Read the model definition and answer for the solid it produces. Units are mm, in the model's axes. Face numbers are marked on the shaded views. A direction names the side the tool comes from. Give positions to 0.01 mm unless a question says otherwise; leave off trailing zeros. Loops run counter-clockwise (first coordinate to the right, second up) from the corner with the lowest first, then second, coordinate; pieces in that order, holes last. Notation, with made-up numbers: (27, 80) - (31, 80) arc R13 cw to (31, 103) - close; hole circle Ø2 at (-2.5, 6.5). An arc over 180 degrees is marked (long way). Put each result on its own line as item: value. Start each with the question number.
1. Consider L1, parallel to Y at x = -8, z = 17.5; L2, parallel to Y at x = 17, z = 20.5; L3, parallel to X at y = 32, z = 5. Determine where each line is inside the solid, lowest interval first. Write a range as from..to.
2. A cutting plane is placed at C-C, the plane y = -9. Determine the outline of the cut face in (x, z), plus the area to 3 significant figures.
3. For a pull along Y with two mould halves and no side action, classify the marked faces 1, 2, 3 and 4 as released by +Y, released by -Y, zero draft, split by the parting line, or undercut.
4. Given pin 1 Ø2.5 at (x, y) = (-11, 4.5) entering from +Z; pin 2 Ø4 at (y, z) = (46, 10) entering from +X; pin 3 Ø8 at (x, z) = (-11.5, 3) entering from +Y; pin 4 Ø5 at (y, z) = (-9.5, 11.5) entering from -X, each flat-ended and moving along its own axis, determine where each tip first touches the part or whether it passes through.
5. A cutting plane is placed at A-A, the plane z = 5. Count the separate pieces of the cut face and the enclosed holes in it, plus the area to 3 significant figures.
6. A cutting plane is placed at B-B, the plane y = 46. Determine the outline of the cut face in (x, z), plus the area to 3 significant figures.
7. For the marked faces 5, 6 and 7, determine the directions among +Z, -Z, +X, -X, +Y, -Y from which every point of the face is accessible in a straight line to the end or side of a thin tool.
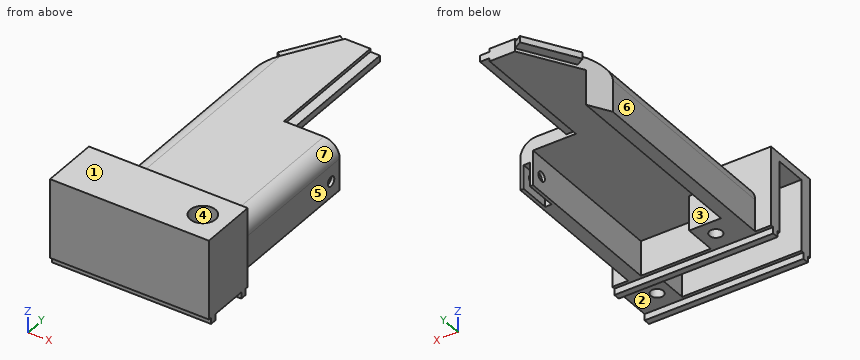
```python
from build123d import *

# Parameters (mm, degrees)
SKETCH1_W                = 40
SKETCH1_H                = 30
BOSS_EXTRUDE1_DEPTH      = 90
SHELL1_T                 = -4
FILLET1_R                = 5
CUT_EXTRUDE1_DEPTH       = 94.407708461
CUT_EXTRUDE1_DEPTH_BACK  = 94.407708461
CUT_EXTRUDE2_DEPTH       = 94.407708461
CUT_EXTRUDE2_DEPTH_BACK  = 94.407708461
SKETCH3_W                = 17.5
SKETCH3_H                = 40
SKETCH5_W                = 2
SKETCH5_H                = 40
BOSS_EXTRUDE2_DEPTH      = 3
SKETCH6_W                = 2
SKETCH6_H                = 18
BOSS_EXTRUDE3_DEPTH      = 3
SKETCH8_W                = 50
SKETCH8_H                = 50
BOSS_EXTRUDE4_DEPTH      = 18
SKETCH10_W               = 45
SKETCH10_H               = 10
CUT_EXTRUDE4_DEPTH       = 37.5
BOSS_EXTRUDE5_REACH      = 103.502
SKETCH15_W               = 10
SKETCH15_H               = 10
CUT_EXTRUDE8_DEPTH       = 103.988587343
CUT_EXTRUDE8_DEPTH_BACK  = 103.988587343
SKETCH20_R               = 2
SKETCH21_R               = 4
CUT_EXTRUDE9_DEPTH       = 5
SKETCH23_W               = 2
SKETCH23_H               = 15
CUT_EXTRUDE10_DEPTH      = 10
CUT_EXTRUDE11_START      = -10
SKETCH24_R               = 1.5
CUT_EXTRUDE11_DEPTH      = 116.031657717
CUT_EXTRUDE12_DEPTH      = 99.140965569
CUT_EXTRUDE12_DEPTH_BACK = 99.140965569
SKETCH27_W               = 50
SKETCH27_H               = 25
SKETCH29_W               = 50
SKETCH29_H               = 2
BOSS_EXTRUDE6_DEPTH      = 2
SKETCH30_W               = 50
SKETCH30_H               = 2
BOSS_EXTRUDE7_DEPTH      = 2
CUT_EXTRUDE13_DEPTH      = 99.66939304
CUT_EXTRUDE13_DEPTH_BACK = 99.66939304
SKETCH31_R               = 2
SKETCH32_R               = 4
CUT_EXTRUDE14_DEPTH      = 15


with BuildPart() as part:
    # Sketch1 → Boss-Extrude1 (new body)
    with BuildSketch(Plane(origin=(0, 0, 0), x_dir=(1, 0, 0), z_dir=(0, 1, 0))):
        Rectangle(SKETCH1_W, SKETCH1_H)
    extrude(amount=BOSS_EXTRUDE1_DEPTH)

    # Shell1
    shell1_openings = [part.faces().sort_by_distance(p)[0] for p in [
        (0, 90, 0),
        (0, 0, 0),
    ]]
    offset(amount=SHELL1_T, openings=shell1_openings, kind=Kind.INTERSECTION)

    # Fillet1
    fillet1_edges = [part.edges().sort_by_distance(p)[0] for p in [
        (20, 45, 15),
        (-20, 45, 15),
        (-20, 45, -15),
        (20, 45, -15),
    ]]
    fillet(fillet1_edges, radius=FILLET1_R)

    # Sketch2 → Cut-Extrude1 (cut, two sides: drawn at the far end of the back side and taken through both)
    with BuildSketch(Plane.XY.offset(-CUT_EXTRUDE1_DEPTH_BACK)):
        Polygon((-5.5, 90), (-20, 66), (-20, 90), align=None)
    extrude(amount=CUT_EXTRUDE1_DEPTH + CUT_EXTRUDE1_DEPTH_BACK, mode=Mode.SUBTRACT)

    # Sketch3 → Cut-Extrude2 (cut, two sides: drawn at the far end of the back side and taken through both)
    with BuildSketch(Plane.XY.offset(-CUT_EXTRUDE2_DEPTH_BACK)):
        with Locations((11.25, 70)):
            Rectangle(SKETCH3_W, SKETCH3_H)
    extrude(amount=CUT_EXTRUDE2_DEPTH + CUT_EXTRUDE2_DEPTH_BACK, mode=Mode.SUBTRACT)

    # Sketch5 → Boss-Extrude2 (add)
    with BuildSketch(Plane(origin=(2.5, 0, 0), x_dir=(0, 0, -1), z_dir=(1, 0, 0))):
        with Locations((-13, 70)):
            Rectangle(SKETCH5_W, SKETCH5_H)
    boss_extrude2 = extrude(amount=BOSS_EXTRUDE2_DEPTH)

    # Mirror1: Boss-Extrude2 across plane
    add(boss_extrude2.mirror(Plane.XY))

    # Sketch6 → Boss-Extrude3 (add)
    with BuildSketch(Plane(origin=(-43.86391097, 26.501112878, 0), x_dir=(0, 0, 1), z_dir=(-0.8559155419457906, 0.5171156399255814, 0))):
        with Locations((-13, 65.188262756)):
            Rectangle(SKETCH6_W, SKETCH6_H)
    boss_extrude3 = extrude(amount=BOSS_EXTRUDE3_DEPTH)

    # Mirror2: Boss-Extrude3 across plane
    add(boss_extrude3.mirror(Plane.XY))

    # Sketch8 → Boss-Extrude4 (add)
    with BuildSketch(Plane(origin=(0, 0, 0), x_dir=(1, 0, 0), z_dir=(0, 1, 0))):
        Rectangle(SKETCH8_W, SKETCH8_H)
    extrude(amount=-BOSS_EXTRUDE4_DEPTH)

    # Sketch10 → Cut-Extrude4 (cut)
    with BuildSketch(Plane.ZY.offset(25)):
        with Locations((0, -9)):
            Rectangle(SKETCH10_W, SKETCH10_H)
    extrude(amount=-CUT_EXTRUDE4_DEPTH, mode=Mode.SUBTRACT)

    # Sketch15 → Boss-Extrude5 (add, up to next)
    with BuildSketch(Plane.XY.offset(-11), mode=Mode.PRIVATE) as boss_extrude5_sk1:
        with Locations((-11, 5)):
            Rectangle(SKETCH15_W, SKETCH15_H)
    boss_extrude5_tool1 = extrude(boss_extrude5_sk1.sketch, amount=BOSS_EXTRUDE5_REACH, mode=Mode.PRIVATE) - part.part
    add(boss_extrude5_tool1.solids().sort_by_distance((-11, 5, -11))[0])

    # Sketch20 → Cut-Extrude8 (cut, two sides: drawn at the far end of the back side and taken through both)
    with BuildSketch(Plane(origin=(0, 0, -15), x_dir=(-1, 0, 0), z_dir=(0, 0, -1)).offset(-CUT_EXTRUDE8_DEPTH_BACK)):
        with Locations((11, 5)):
            Circle(SKETCH20_R)
    extrude(amount=CUT_EXTRUDE8_DEPTH + CUT_EXTRUDE8_DEPTH_BACK, mode=Mode.SUBTRACT)

    # Sketch21 → Cut-Extrude9 (cut)
    with BuildSketch(Plane(origin=(0, 0, -15), x_dir=(-1, 0, 0), z_dir=(0, 0, -1))):
        with Locations((11, 5)):
            Circle(SKETCH21_R)
    cut_extrude9 = extrude(amount=-CUT_EXTRUDE9_DEPTH, mode=Mode.SUBTRACT)

    # Mirror3: Cut-Extrude9 across plane
    add(cut_extrude9.mirror(Plane.XY), mode=Mode.SUBTRACT)

    # Sketch23 → Cut-Extrude10 (cut)
    with BuildSketch(Plane(origin=(0, 50, 0), x_dir=(1, 0, 0), z_dir=(0, 1, 0))):
        with Locations((17.949489743, 0)):
            Rectangle(SKETCH23_W, SKETCH23_H)
    extrude(amount=-CUT_EXTRUDE10_DEPTH, mode=Mode.SUBTRACT)

    # Sketch24 → Cut-Extrude11 (cut)
    with BuildSketch(Plane(origin=(20, 0, 0), x_dir=(0, 0, -1), z_dir=(1, 0, 0)).offset(CUT_EXTRUDE11_START)):
        with Locations(Location((-5, 46, 0), (0, 0, 180))):
            Circle(SKETCH24_R)
    cut_extrude11 = extrude(amount=CUT_EXTRUDE11_DEPTH, mode=Mode.SUBTRACT)

    # Mirror4: Cut-Extrude11 across plane
    add(cut_extrude11.mirror(Plane.XY), mode=Mode.SUBTRACT)

    # Sketch27 → Cut-Extrude12 (cut, two sides: drawn at the far end of the back side and taken through both)
    with BuildSketch(Plane(origin=(0, 0, 0), x_dir=(1, 0, 0), z_dir=(0, 1, 0)).offset(-CUT_EXTRUDE12_DEPTH_BACK)):
        with Locations((0, 12.5)):
            Rectangle(SKETCH27_W, SKETCH27_H)
    extrude(amount=CUT_EXTRUDE12_DEPTH + CUT_EXTRUDE12_DEPTH_BACK, mode=Mode.SUBTRACT)

    # Sketch29 → Boss-Extrude6 (add)
    with BuildSketch(Plane(origin=(0, 0, 0), x_dir=(-1, 0, 0), z_dir=(0, 0, -1))):
        with Locations((0, -2)):
            Rectangle(SKETCH29_W, SKETCH29_H)
    extrude(amount=BOSS_EXTRUDE6_DEPTH)

    # Sketch30 → Boss-Extrude7 (add)
    with BuildSketch(Plane(origin=(0, 0, 0), x_dir=(-1, 0, 0), z_dir=(0, 0, -1))):
        with Locations((0, -16)):
            Rectangle(SKETCH30_W, SKETCH30_H)
    extrude(amount=BOSS_EXTRUDE7_DEPTH)

    # Sketch31 → Cut-Extrude13 (cut, two sides: drawn at the far end of the back side and taken through both)
    with BuildSketch(Plane.XY.offset(25).offset(-CUT_EXTRUDE13_DEPTH_BACK)):
        with Locations((17, -9)):
            Circle(SKETCH31_R)
    extrude(amount=CUT_EXTRUDE13_DEPTH + CUT_EXTRUDE13_DEPTH_BACK, mode=Mode.SUBTRACT)

    # Sketch32 → Cut-Extrude14 (cut)
    with BuildSketch(Plane.XY.offset(25)):
        with Locations((17, -9)):
            Circle(SKETCH32_R)
    extrude(amount=-CUT_EXTRUDE14_DEPTH, mode=Mode.SUBTRACT)


solid = part.part
```
Return value:
1. L1: y = -18..-14, -4..0
1. L2: y = -18..-13, -5..0
1. L3: x = -20..-16, 16..20
2. outline: (-25, 22.5) - (12.5, 22.5) - (12.5, 0) - (15, 0) - (15, 10) - (13, 10) - (13, 25) - (-25, 25) - close; (19, 0) - (25, 0) - (25, 25) - (21, 25) - (21, 10) - (19, 10) - close
2. area: 246 mm2
3. face 1: zero draft
3. face 2: undercut
3. face 3: released by +Y
3. face 4: undercut
4. pin 1: passes through
4. pin 2: stops at x = 20
4. pin 3: stops at y = 10
4. pin 4: stops at x = 12.5
5. separate pieces: 3
5. enclosed holes: 2
5. area: 1,050 mm2
6. outline: (-20, 0) - (-16, 0) - (-16, 11) - (16, 11) - (16, 6.5) - (16.95, 6.5) - (16.95, 7.5) - (18.95, 7.5) - (18.95, 6.5) - (20, 6.5) - (20, 10) arc R5 ccw to (15, 15) - (-15, 15) arc R5 ccw to (-20, 10) - close; (16, 0) - (16.95, 0) - (16.95, 3.5) - (16, 3.5) - close; (18.95, 0) - (20, 0) - (20, 3.5) - (18.95, 3.5) - close
6. area: 216 mm2
7. face 5: +Z, -Z, +X, +Y
7. face 6: +Z, -Z, -X, +Y
7. face 7: +Z, +X, +Y
